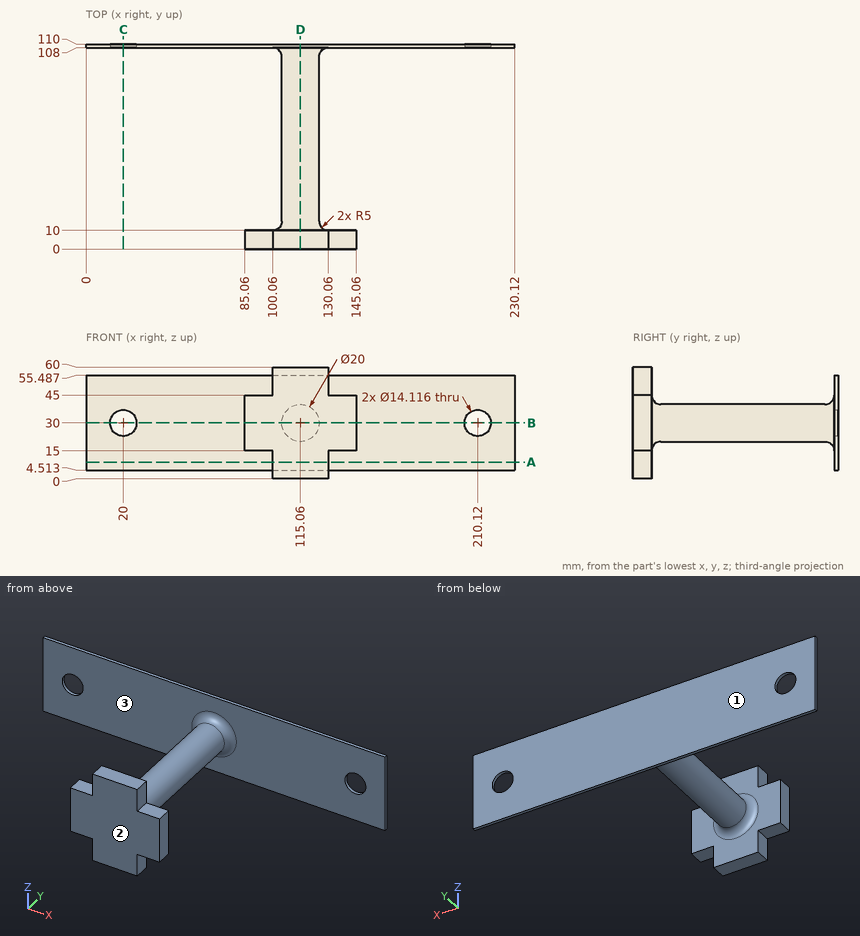
Source: three-view drawing plus pictorial views. Frame: mm from the lowest corner of the part. Coordinates: 2 decimals unless noted, no trailing zeros. Loops run counter-clockwise (first coordinate to the right, second up) from the corner with the lowest first, then second, coordinate; pieces in that order, holes last. Notation, with made-up numbers: (39.25, 53) - (80.25, 53) arc R22 cw to (80.25, 81) - close; hole circle Ø9 at (8.25, 89). An arc over 180 degrees is marked (long way). One line per item, written item: value. Start each with the question number.
1. Section C-C (x = 20). Return the cut outline in (y, z).
2. Mould query, pull axis Y, two halves, no side actions, for the marked faces 1, 2 and 3. Classes: pulls with the +Y half, pulls with the -Y half, needs draft (parallel to the pull), parting line crosses it, or undercut.
3. Section A-A (z = 9). Return the cut outline in (x, y).
4. Contact query for flat-ended pins moving along their axis: P1, Ø5, axis at x = 89.5, y = 4.5, coming from the +Z side; P2, Ø0.6, axis at x = 169.5, y = 109, coming from the -Z side; P3, Ø8, axis at x = 96, y = 5, coming from the -Z side. Output: stop coordinate, or through.
5. Section D-D (x = 115.06). Return the cut outline in (y, z), and give its area (3 significant figures).
6. Section B-B (z = 30). Return the cut outline in (x, y).
7. Ray query, L1, parallel to X at y = 109.25, z = 30; L2, parallel to Y at x = 97, z = 44.5; L3, parallel to Y at x = 208.5, z = 41.5. Return the intervals inside material, ascending.
Verdict:
1. outline: (108, 4.51) - (110, 4.51) - (110, 22.94) - (108, 22.94) - close; (108, 37.06) - (110, 37.06) - (110, 55.49) - (108, 55.49) - close
2. face 1: pulls with the +Y half
2. face 2: pulls with the -Y half
2. face 3: undercut
3. outline: (0, 108) - (230.12, 108) - (230.12, 110) - (0, 110) - close; (100.06, 0) - (130.06, 0) - (130.06, 10) - (100.06, 10) - close
4. P1: stops at z = 45
4. P2: stops at z = 4.51
4. P3: stops at z = 15
5. outline: (0, 0) - (10, 0) - (10, 15) arc R5 cw to (15, 20) - (103, 20) arc R5 cw to (108, 15) - (108, 4.51) - (110, 4.51) - (110, 55.49) - (108, 55.49) - (108, 45) arc R5 cw to (103, 40) - (15, 40) arc R5 cw to (10, 45) - (10, 60) - (0, 60) - close
5. area: 2,680 mm2
6. outline: (0, 108) - (12.94, 108) - (12.94, 110) - (0, 110) - close; (27.06, 108) - (100.06, 108) arc R5 cw to (105.06, 103) - (105.06, 15) arc R5 cw to (100.06, 10) - (85.06, 10) - (85.06, 0) - (145.06, 0) - (145.06, 10) - (130.06, 10) arc R5 cw to (125.06, 15) - (125.06, 103) arc R5 cw to (130.06, 108) - (203.06, 108) - (203.06, 110) - (27.06, 110) - close; (217.18, 108) - (230.12, 108) - (230.12, 110) - (217.18, 110) - close
7. L1: x = 0 to 12.94, 27.06 to 203.06, 217.18 to 230.12
7. L2: y = 0 to 10, 108 to 110
7. L3: y = 108 to 110
